from build123d import *

# Parameters (mm, degrees)
BOSS_EXTRUDE1_DEPTH = 20
M5_TAPPED_HOLE1_D   = 4.2


with BuildPart() as part:
    # Sketch1 → Boss-Extrude1 (new body)
    with BuildSketch(Plane(origin=(0, 0, 0), x_dir=(0, 0, -1), z_dir=(1, 0, 0))):
        Polygon((0, 0), (0, 62), (6.35, 62), (6.35, 6.35), (20, 6.35), (20, 0), align=None)
    extrude(amount=BOSS_EXTRUDE1_DEPTH)

    # M5 Tapped Hole1 (through all)
    with Locations(Plane.XY):
        with Locations((10, 52)):
            Hole(M5_TAPPED_HOLE1_D / 2)


solid = part.part
Work out the finished part from the listing and answer in its coordinate system (mm). A direction names the side the tool comes from. Coordinates: 2 decimals unless noted, no trailing zeros. Write each loop counter-clockwise with the first axis right and the second up, starting at its lowest first coordinate (ties: lowest second). Pieces come first, ordered by that corner, then holes. Notation, with made-up numbers: M 29,87.25 L 57,87.25 A22 ccw 57,96.25 Z; hole C 64.5,5.5 d4. An arc over 180 degrees is marked long. Answer as CSV lines item,"result". Start each with the question number.
Item 1: Consider L1, parallel to Y at x = 10, z = -2.25; L2, parallel to Y at x = 15.25, z = -10.25; L3, parallel to Z at x = 16.5, y = 16. Determine where each line is inside the solid, lowest interval first.
Item 2: Flat-ended cylindrical pins translate along their axes: P1, Ø10, axis at x = 16.5, y = 31.5, coming from the +Z side; P2, Ø1.5, axis at x = 11, y = 13, coming from the -Z side; P3, Ø11, axis at x = 10.5, z = -13.5, coming from the +Y side. Find the tip coordinate at first contact, or state that the pin passes through.
Item 3: A tool of negligible diameter and unlimited length cuts with its end or side. For faces 4 (the face through (10, 3, -20)), 5 (the face through (10, 6.35, -13)), from which of +Z, -Z, +X, -X, +Y, -Y can it reach the whole face along a straight path? Write none if from no direction.
Item 4: Section B-B on y = 52 is taken. Write down the section's boundary in (x, z), and give its area (3 significant figures).
Item 5: Section A-A on x = 10 is taken. Write down the section's boundary in (y, z), and give its area (3 significant figures).
Item 6: Determine the mould class of faces 1 (the face through (20, 25, -6)), 2 (the face through (10, 0, -10)), 3 (the face through (11.666, 50.722, -3.219)) for opening direction X: released by +X, released by -X, zero draft, split by the parting line, or undercut.
Item 7: Section C-C on y = 9 is taken. Write down the section's boundary in (x, z), and give its area (3 significant figures).
Item 8: Section D-D on z = -18 is taken. Write down the section's boundary in (x, y), and give its area (3 significant figures).
Checks:
1,L1,"y = 0 to 49.9, 54.1 to 62"
1,L2,"y = 0 to 6.35"
1,L3,"z = -6.35 to 0"
2,P1,"stops at z = 0"
2,P2,"stops at z = -6.35"
2,P3,"stops at y = 6.35"
3,face 4,"-Z, +X, -X, +Y, -Y"
3,face 5,"-Z, +X, -X, +Y"
4,outline,"M 0,-6.35 L 7.9,-6.35 L 7.9,0 L 0,0 Z; M 12.1,-6.35 L 20,-6.35 L 20,0 L 12.1,0 Z"
4,area,"100 mm²"
5,outline,"M 0,-20 L 6.35,-20 L 6.35,-6.35 L 49.9,-6.35 L 49.9,0 L 0,0 Z; M 54.1,-6.35 L 62,-6.35 L 62,0 L 54.1,0 Z"
5,area,"454 mm²"
6,face 1,"released by +X"
6,face 2,"zero draft"
6,face 3,"undercut"
7,outline,"M 0,-6.35 L 20,-6.35 L 20,0 L 0,0 Z"
7,area,"127 mm²"
8,outline,"M 0,0 L 20,0 L 20,6.35 L 0,6.35 Z"
8,area,"127 mm²"
